Can you work these out from the model? Positions are in its coordinate system, mm. Face numbers are marked on the shaded views. A direction names the side the tool comes from. Coordinates: 2 decimals unless noted, no trailing zeros. Order: outer loops, then holes, each group sorted by start corner. A loop starts at its lowest first (then second) coordinate and runs counter-clockwise, first axis right, second up. Notation, with made-up numbers: (-14, -5) -> (17, -5) arc R16 cw to (17, 14) -> close; hole circle Ø11 at (40.25, 45). An arc over 180 degrees is marked (long way). Use a Markdown table: item, result. Add a question column.
1. If I drill on line 1 along Y through (x, z) = (-17, 2.5); line 2 along Z through (x, y) = (0, -3); line 3 along X through (y, z) = (0, 3.75), over which ranges is the centre line in solid material (lowest first)? Write a range as from..to.
2. Suppose I cut it at A-A, the plane y = 0. List the corners of the cut face in (x, z) for me.
3. We'd pull the mould along Y, two halves only. Please class the marked faces 1, 2, 3 and 4: pulls with the +Y half, pulls with the -Y half, needs draft (parallel to the pull), parting line crosses it, or undercut.
4. For the marked faces 5 and 6, which set-ups out of +Z, -Z, +X, -X, +Y, -Y let a thin tool reach every point of the face, with its end or its side?
5. For pin 1 Ø2.5 at (x, z) = (0, 0) entering from +Y; pin 2 Ø5 at (x, z) = (-13.5, 0) entering from -Y, each with a flat end and sliding along its axis, tell me the tip position at first contact or that it passes through.
6. Suppose I cut it at D-D, the plane y = 3.75. List the corners of the cut face in (x, z) for me, then the cut area to 3 significant figures.
7. Suppose I cut it at C-C, the plane x = 0. List the corners of the cut face in (y, z) for me.
8. Suppose I cut it at B-B, the plane z = 0. List the corners of the cut face in (x, y) for me.
```python
from build123d import *

# Parameters (mm, degrees)
F0_W     = 50
F0_H     = 10
F0_R     = 1.9
F1_DEPTH = 5
F2_SIZE  = 1
F4_DEPTH = 12.5
F5_R     = 3
F5_R_2   = 1.9
F6_DEPTH = 2


# Not quite as in the source:
# - a feature names something its author has since deleted; it is built from what else it names


with BuildPart() as f1:
    # F0 (on Front) → F1 (new body, symmetric)
    with BuildSketch(Plane.XZ):
        Rectangle(F0_W, F0_H)
        Circle(F0_R, mode=Mode.SUBTRACT)
    extrude(amount=F1_DEPTH, both=True)

    # F2
    f2_edges = [f1.edges().sort_by_distance(p)[0] for p in [
        (-25, 0, -5),
        (25, 0, -5),
    ]]
    chamfer(f2_edges, length=F2_SIZE)

    # F3 (on Top) → F4 (cut, symmetric)
    with BuildSketch(Plane.XY):
        with BuildLine():
            ThreePointArc((-20, 1.85), (-21.85, 0), (-20, -1.85))
            Line((-20, -1.85), (-5, -1.85))
            ThreePointArc((-5, -1.85), (-3.15, 0), (-5, 1.85))
            Line((-5, 1.85), (-20, 1.85))
        make_face()
        with BuildLine():
            Line((5, -1.85), (20, -1.85))
            ThreePointArc((20, -1.85), (21.85, 0), (20, 1.85))
            Line((20, 1.85), (5, 1.85))
            ThreePointArc((5, 1.85), (3.15, 0), (5, -1.85))
        make_face()
    extrude(amount=F4_DEPTH, both=True, mode=Mode.SUBTRACT)

    # F5 (on face) → F6 (join)
    with BuildSketch(Plane.XZ.offset(5)):
        Circle(F5_R)
        Circle(F5_R_2, mode=Mode.SUBTRACT)
    extrude(amount=F6_DEPTH)


solid = f1.part
```
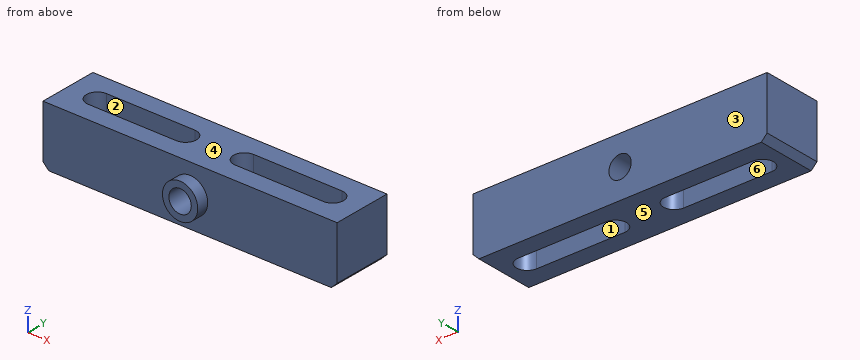
Worked out:
| question | item | result |
|---|---|---|
| 1 | line 1 | y = -5..-1.85, 1.85..5 |
| 1 | line 2 | z = -5..-1.9, 1.9..5 |
| 1 | line 3 | x = -25..-21.85, -3.15..3.15, 21.85..25 |
| 2 | outline | (-25, -4) -> (-24, -5) -> (-21.85, -5) -> (-21.85, 5) -> (-25, 5) -> close; (-3.15, -5) -> (3.15, -5) -> (3.15, 5) -> (-3.15, 5) -> close; (21.85, -5) -> (24, -5) -> (25, -4) -> (25, 5) -> (21.85, 5) -> close; hole circle Ø3.8 at (0, 0) |
| 3 | face 1 | undercut |
| 3 | face 2 | undercut |
| 3 | face 3 | pulls with the +Y half |
| 3 | face 4 | needs draft |
| 4 | face 5 | -Z, +X, -X, +Y, -Y |
| 4 | face 6 | +Z, -Z |
| 5 | pin 1 | passes through |
| 5 | pin 2 | stops at y = -5 |
| 6 | outline | (-25, -4) -> (-24, -5) -> (24, -5) -> (25, -4) -> (25, 5) -> (-25, 5) -> close; hole circle Ø3.8 at (0, 0) |
| 6 | area | 488 mm² |
| 7 | outline | (-7, -3) -> (-5, -3) -> (-5, -5) -> (5, -5) -> (5, -1.9) -> (-7, -1.9) -> close; (-7, 1.9) -> (5, 1.9) -> (5, 5) -> (-5, 5) -> (-5, 3) -> (-7, 3) -> close |
| 8 | outline | (-25, -5) -> (-3, -5) -> (-3, -7) -> (-1.9, -7) -> (-1.9, 5) -> (-25, 5) -> close; (1.9, -7) -> (3, -7) -> (3, -5) -> (25, -5) -> (25, 5) -> (1.9, 5) -> close; hole (-20, -1.85) -> (-5, -1.85) arc R1.85 ccw to (-5, 1.85) -> (-20, 1.85) arc R1.85 ccw to start; hole (5, -1.85) -> (20, -1.85) arc R1.85 ccw to (20, 1.85) -> (5, 1.85) arc R1.85 ccw to start |
